Could you check a few things on this model? Use its own coordinates, in mm. Face numbers are marked on the shaded views. A direction names the side the tool comes from. Give positions to 0.01 mm unless a question says otherwise; leave off trailing zeros. Order: outer loops, then holes, each group sorted by start corner. A loop starts at its lowest first (then second) coordinate and runs counter-clockwise, first axis right, second up. Notation, with made-up numbers: M -7.75,75 L 2.25,75 A19 ccw 2.25,81 Z; hole C -17,-6 d3. An arc over 180 degrees is marked long. Use a Markdown table: item, result. Add a question column.
Item 1: If we mould it in two halves opening along X, with no side actions, what happens to the marked faces 4, 5 and 6? For each: released by +X, released by -X, zero draft, split by the parting line, or undercut.
Item 2: For the marked faces 1, 2 and 3, which set-ups out of +Z, -Z, +X, -X, +Y, -Y let a thin tool reach every point of the face, with its end or its side?
Item 3: I'm going to push flat-ended pins straight in: pin 1 Ø2 at (x, y) = (31, -5) entering from +Z; pin 2 Ø2 at (x, y) = (6.5, -3.5) entering from -Z; pin 3 Ø2.5 at (y, z) = (-3.5, -2) entering from +X; pin 4 Ø4 at (x, z) = (-1.5, -0.5) entering from +Y. Where does each tip first touch, or does it pass through?
Item 4: Suppose I cut it at D-D on y = -7. Write out the boundary of the cut face in (x, z), plus the area to 3 significant figures.
Item 5: Suppose I cut it at B-B on x = -15. Write out the boundary of the cut face in (y, z).
Item 6: Suppose I cut it at C-C on z = 0. Write out the boundary of the cut face in (x, y), plus the area to 3 significant figures.
Item 7: Suppose I cut it at A-A on y = -1.25. Write out the boundary of the cut face in (x, z), plus the area to 3 significant figures.
Item 8: If I drill on L1, parallel to Z at x = 15, y = -3.5; L2, parallel to X at y = -2.5, z = -4; L3, parallel to Y at x = 4.5, z = 3.75, over which ranges is the centre line in solid material (lowest first)? Write a range as from..to.
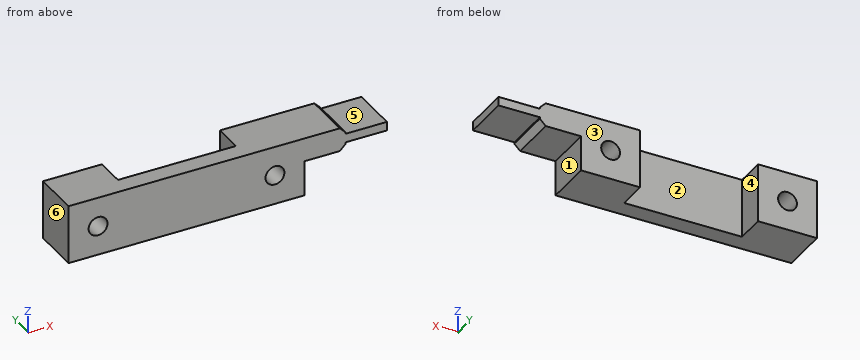
from build123d import *

# Parameters (mm, degrees)
F0_W      = 40
F0_H      = 10
F1_DEPTH  = 8
F2_W      = 20
F2_H      = 5
F3_DEPTH  = 10
F4_R      = 1.6
F5_R      = 1.6
F6_DEPTH  = 8
F7_W      = 8
F7_H      = 4
F8_DEPTH  = 7
F9_W      = 8
F9_H      = 1.5
F10_DEPTH = 7
F11_SIZE  = 1


with BuildPart() as f1:
    # F0 (on Front) → F1 (new body)
    with BuildSketch(Plane.XZ):
        Rectangle(F0_W, F0_H)
    extrude(amount=F1_DEPTH)

    # F2 (on face) → F3 (cut, through all)
    with BuildSketch(Plane.XY.offset(5)):
        with Locations((0, -2.5)):
            Rectangle(F2_W, F2_H)
    extrude(amount=-F3_DEPTH, mode=Mode.SUBTRACT)

    # F4 (on face) + F5 (on face) → F6 (cut, through all)
    with BuildSketch(Plane(origin=(0, 0, 0), x_dir=(-1, 0, 0), z_dir=(0, 1, 0))):
        with Locations((-15, 0)):
            Circle(F4_R)
    with BuildSketch(Plane(origin=(0, 0, 0), x_dir=(-1, 0, 0), z_dir=(0, 1, 0))):
        with Locations((15, 0)):
            Circle(F5_R)
    extrude(amount=-F6_DEPTH, mode=Mode.SUBTRACT)

    # F7 (on face) → F8 (join)
    with BuildSketch(Plane.YZ.offset(20)):
        with Locations((-4, 3)):
            Rectangle(F7_W, F7_H)
    extrude(amount=F8_DEPTH)

    # F9 (on face) → F10 (join)
    with BuildSketch(Plane.YZ.offset(27)):
        with Locations((-4, 3)):
            Rectangle(F9_W, F9_H)
    extrude(amount=F10_DEPTH)

    # F11
    f11_edges = [f1.edges().sort_by_distance(p)[0] for p in [
        (27, -4, 1),
        (27, -4, 5),
    ]]
    chamfer(f11_edges, length=F11_SIZE)


solid = f1.part
Findings below:
| question | item | result |
|---|---|---|
| 1 | face 4 | undercut |
| 1 | face 5 | zero draft |
| 1 | face 6 | released by -X |
| 2 | face 1 | -Z, +X, +Y, -Y |
| 2 | face 2 | +Z, -Z, +Y |
| 2 | face 3 | +Z, -Z, +X, -X, +Y |
| 3 | pin 1 | stops at z = 3.75 |
| 3 | pin 2 | passes through |
| 3 | pin 3 | stops at x = 20 |
| 3 | pin 4 | stops at y = -5 |
| 4 | outline | M -20,-5 L 20,-5 L 20,1 L 26,1 L 27,2 L 27,2.25 L 34,2.25 L 34,3.75 L 27,3.75 L 27,4 L 26,5 L -20,5 Z; hole C -15,0 d3.2; hole C 15,0 d3.2 |
| 4 | area | 421 mm^2 |
| 5 | outline | M -8,-5 L 0,-5 L 0,-1.6 L -8,-1.6 Z; M -8,1.6 L 0,1.6 L 0,5 L -8,5 Z |
| 6 | outline | M -20,-8 L -16.6,-8 L -16.6,0 L -20,0 Z; M -13.4,-8 L 13.4,-8 L 13.4,0 L 10,0 L 10,-5 L -10,-5 L -10,0 L -13.4,0 Z; M 16.6,-8 L 20,-8 L 20,0 L 16.6,0 Z |
| 6 | area | 169 mm^2 |
| 7 | outline | M -20,-5 L -10,-5 L -10,5 L -20,5 Z; M 10,-5 L 20,-5 L 20,1 L 26,1 L 27,2 L 27,2.25 L 34,2.25 L 34,3.75 L 27,3.75 L 27,4 L 26,5 L 10,5 Z; hole C -15,0 d3.2; hole C 15,0 d3.2 |
| 7 | area | 221 mm^2 |
| 8 | L1 | z = -5..-1.6, 1.6..5 |
| 8 | L2 | x = -20..-10, 10..20 |
| 8 | L3 | y = -8..-5 |
